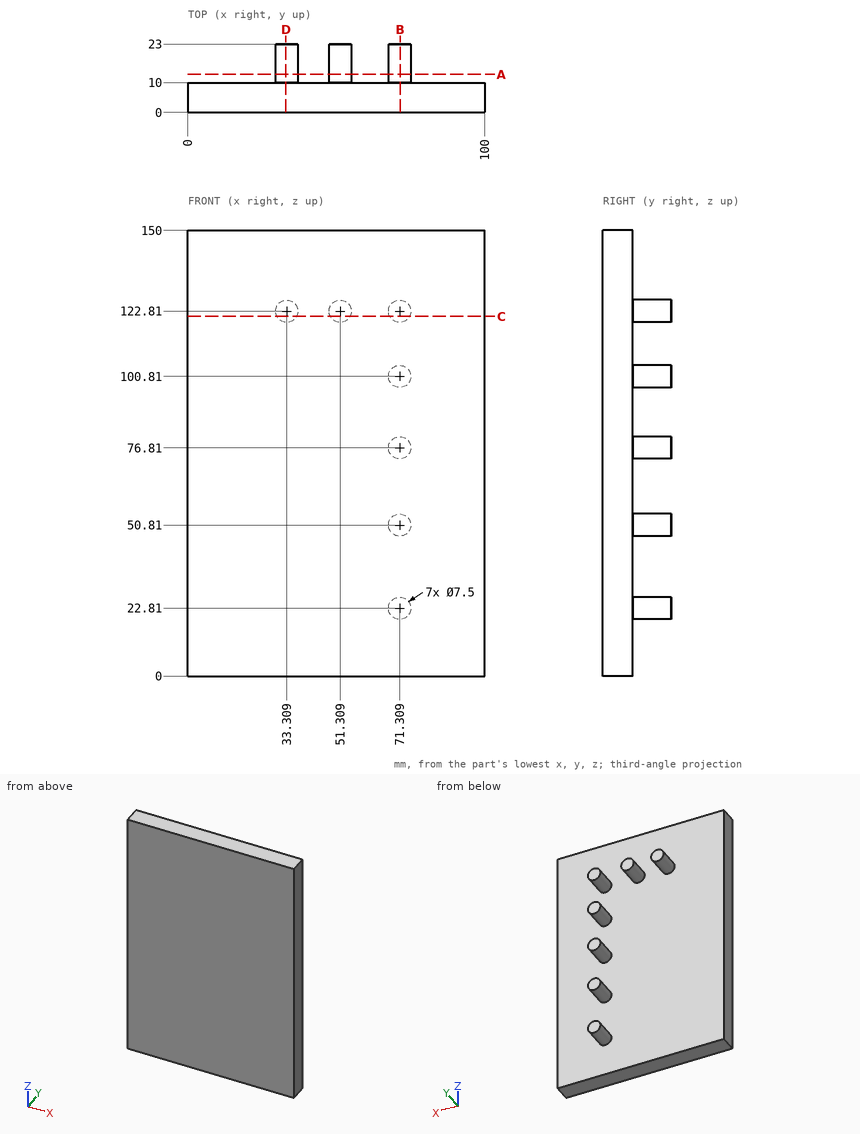
Geometry: see drawing. Coordinates: mm, zero at the bounding-box minimum. Round coordinates to 2 decimals unless told otherwise and drop trailing zeros. Write each loop counter-clockwise with the first axis right and the second up, starting at its lowest first coordinate (ties: lowest second). Pieces come first, ordered by that corner, then holes.
1) Ray query, L1, parallel to X at y = 15, z = 121.5 (1 decimal); L2, parallel to Y at x = 50, z = 31.5; L3, parallel to X at y = 16.25, z = 24 (1 decimal). Return the intervals inside material, ascending.
2) Cut plane A-A (y = 12.75). Return the cut outline in (x, z).
3) Cut plane D-D (x = 33). Return the cut outline in (y, z).
4) Cut plane C-C (z = 121). Return the cut outline in (x, y) (1 decimal), then the cut area to 3 significant figures.
5) Cut plane B-B (x = 71.5). Return the cut outline in (y, z) (1 decimal), then the cut area to 3 significant figures.
6) Contact query for flat-ended pins moving along their axis: P1, Ø1, axis at x = 69, y = 7.5, coming from the -Z side; P2, Ø5, axis at x = 18, z = 61, coming from the +Y side; P3, Ø1.5, axis at x = 21.5, y = 12.5, coming from the -Z side. Output: stop coordinate, or through.
Geometry says:
1. L1: x = 29.8 to 36.8, 47.8 to 54.8, 67.8 to 74.8
1. L2: y = 0 to 10
1. L3: x = 67.8 to 74.9
2. outline: circle Ø7.5 at (33.31, 122.81); circle Ø7.5 at (51.31, 122.81); circle Ø7.5 at (71.31, 22.81); circle Ø7.5 at (71.31, 50.81); circle Ø7.5 at (71.31, 76.81); circle Ø7.5 at (71.31, 100.81); circle Ø7.5 at (71.31, 122.81)
3. outline: (0, 0) - (10, 0) - (10, 119.07) - (23, 119.07) - (23, 126.55) - (10, 126.55) - (10, 150) - (0, 150) - close
4. outline: (0, 0) - (100, 0) - (100, 10) - (74.6, 10) - (74.6, 23) - (68, 23) - (68, 10) - (54.6, 10) - (54.6, 23) - (48, 23) - (48, 10) - (36.6, 10) - (36.6, 23) - (30, 23) - (30, 10) - (0, 10) - close
4. area: 1,260 mm2
5. outline: (0, 0) - (10, 0) - (10, 19.1) - (23, 19.1) - (23, 26.6) - (10, 26.6) - (10, 47.1) - (23, 47.1) - (23, 54.6) - (10, 54.6) - (10, 73.1) - (23, 73.1) - (23, 80.6) - (10, 80.6) - (10, 97.1) - (23, 97.1) - (23, 104.6) - (10, 104.6) - (10, 119.1) - (23, 119.1) - (23, 126.6) - (10, 126.6) - (10, 150) - (0, 150) - close
5. area: 1,990 mm2
6. P1: stops at z = 0
6. P2: stops at y = 10
6. P3: passes through
